CAD build for the part. Positions are in the model's coordinates, mm. Face numbers are marked on the shaded views. A direction names the side the tool comes from. Round coordinates to 2 decimals unless told otherwise and drop trailing zeros. Write each loop counter-clockwise with the first axis right and the second up, starting at its lowest first coordinate (ties: lowest second). Pieces come first, ordered by that corner, then holes. Notation, with made-up numbers: M 76.5,71.25 L 107.5,71.25 A8 cw 107.5,80.25 Z; hole C 71,78 d7. An arc over 180 degrees is marked long. Write each question's results on one line, items separated by ' | '. Start each with the question number.
```python
from build123d import *

# Parameters (mm, degrees)
BOSS_EXTRUDE1_DEPTH     = 38.735
SHELL1_T                = -2.54
SKETCH4_W               = 35.167060632
SKETCH4_H               = 72.39
CUT_EXTRUDE1_DEPTH      = 87.281603677
CUT_EXTRUDE2_DEPTH      = 111.946262659
CUT_EXTRUDE2_DEPTH_BACK = 111.946262659
SKETCH6_R               = 3.175


with BuildPart() as part:
    # Sketch1 → Boss-Extrude1 (new, symmetric)
    with BuildSketch(Plane.XY):
        Polygon((-19.05, 0), (19.05, 0), (31.75, 21.997045256), (31.75, 72.797045256), (-31.75, 72.797045256), (-31.75, 21.997045256), align=None)
    extrude(amount=BOSS_EXTRUDE1_DEPTH, both=True)

    # Shell1
    shell1_openings = [part.faces().sort_by_distance(p)[0] for p in [
        (0, 72.797045256, 0),
    ]]
    offset(amount=SHELL1_T, openings=shell1_openings, kind=Kind.INTERSECTION)

    # Sketch4 → Cut-Extrude1 (cut, through all)
    with BuildSketch(Plane(origin=(0, 2.54, 0), x_dir=(1, 0, 0), z_dir=(0, 1, 0))):
        Rectangle(SKETCH4_W, SKETCH4_H)
    extrude(amount=-CUT_EXTRUDE1_DEPTH, mode=Mode.SUBTRACT)

    # Sketch6 → Cut-Extrude2 (cut, two sides: drawn at the far end of the back side and taken through both)
    with BuildSketch(Plane.XY.offset(38.735).offset(-CUT_EXTRUDE2_DEPTH_BACK)):
        with Locations((0, 21.997045256)):
            Circle(SKETCH6_R)
    extrude(amount=CUT_EXTRUDE2_DEPTH + CUT_EXTRUDE2_DEPTH_BACK, mode=Mode.SUBTRACT)


solid = part.part
```
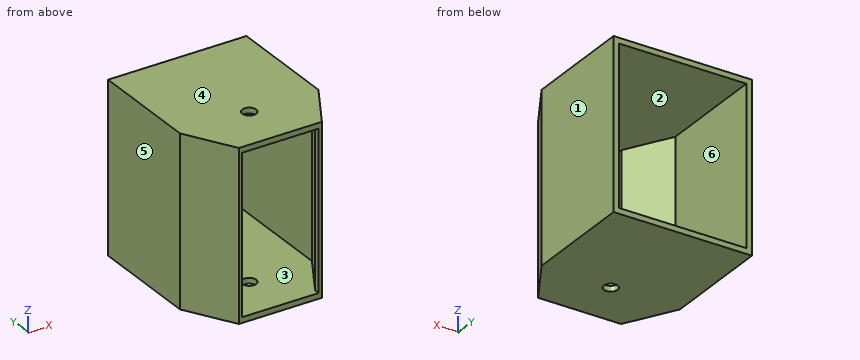
1) Pull direction X, two halves, no side cores. Call the marked faces 3, 4, 5 and 6: pulls with the +X half, pulls with the -X half, needs draft (parallel to the pull), parting line crosses it, or undercut.
2) 3-axis set-ups, long thin cutter, end or side, ignore diameter. For the marked faces 1 and 2: which of +Z, -Z, +X, -X, +Y, -Y reach the whole face in a straight line?
3) Saw through at D-D, the plane y = 8. Write the cut outline in (x, z) (3 decimals), plus the area to 3 significant figures.
4) Saw through at A-A, the plane z = -20.5. Write the cut outline in (x, y), plus the area to 3 significant figures.
5) Wall check: line 1 along X through (y, z) = (55, -1.5); line 2 along Z through (x, y) = (14, 28) (3 decimals); line 3 along Y through (x, z) = (0, -37). Give the ranges that are in metal, low to high. Write a range as from..to.
6) Saw through at C-C, the plane y = 52.5. Write the cut outline in (x, z) (3 decimals).
7) Drop flat-ended pins along their axis: pin 1 Ø4 at (x, y) = (0, 22) entering from -Z; pin 2 Ø6 at (y, z) = (12, -12) entering from -X; pin 3 Ø8 at (x, z) = (14, -24.5) entering from +Y; pin 4 Ø8 at (x, z) = (15.5, 15) entering from +Y. Give the stop position or say it passes through.
8) Saw through at B-B, the plane x = -6. Write the cut outline in (y, z) (3 decimals), plus the area to 3 significant figures.
Filled sheet:
1) face 3: undercut | face 4: needs draft | face 5: pulls with the -X half | face 6: undercut
2) face 1: +Z, -Z, +X, +Y, -Y | face 2: +Y
3) outline: M -23.669,-38.735 L 23.669,-38.735 L 23.669,38.735 L -23.669,38.735 Z; hole M -20.736,-36.195 L 20.736,-36.195 L 20.736,36.195 L -20.736,36.195 Z | area: 665 mm^2
4) outline: M -31.75,22 L -19.05,0 L -17.58,0 L -17.58,2.54 L -29.21,22.68 L -29.21,72.8 L -31.75,72.8 Z; M 17.58,0 L 19.05,0 L 31.75,22 L 31.75,72.8 L 29.21,72.8 L 29.21,22.68 L 17.58,2.54 Z | area: 384 mm^2
5) line 1: x = -31.75..-29.21, 29.21..31.75 | line 2: z = -38.735..-36.195, 36.195..38.735 | line 3: y = 0..18.82, 25.17..72.8
6) outline: M -31.75,-38.735 L 31.75,-38.735 L 31.75,38.735 L -31.75,38.735 Z; hole M -29.21,-36.195 L 29.21,-36.195 L 29.21,36.195 L -29.21,36.195 Z
7) pin 1: passes through | pin 2: stops at x = -27.71 | pin 3: stops at y = 3.26 | pin 4: stops at y = 5.86
8) outline: M 0,-38.735 L 72.797,-38.735 L 72.797,-36.195 L 0,-36.195 Z; M 0,36.195 L 72.797,36.195 L 72.797,38.735 L 0,38.735 Z | area: 370 mm^2
